Source: CAD feature listing. Evaluate the final solid. Frame: model axes, mm. A direction names the side the tool comes from. Round coordinates to 2 decimals unless told otherwise and drop trailing zeros. Loops run counter-clockwise (first coordinate to the right, second up) from the corner with the lowest first, then second, coordinate; pieces in that order, holes last. Notation, with made-up numbers: M 15,65 L 59,65 A10 ccw 59,71 Z; hole C 6.5,-37 d11. An arc over 180 degrees is marked long. One line per item, written item: value.
from build123d import *

# Parameters (mm, degrees)
SKETCH_1_W                      = 70
SKETCH_1_H                      = 105
EXTRUDE_1_DEPTH                 = 5
SKETCH_2_W                      = 30
SKETCH_2_H                      = 30
EXTRUDE_2_DEPTH                 = 120
EXTRUDE_3_REACH                 = 137.577
EXTRUDE_3_DIRECTION_2_REACH     = 137.577
SKETCH_8_R                      = 4.1
CUT_EXTRUDE_2_DEPTH             = 5
SKETCH_11_W                     = 20
SKETCH_11_H                     = 105
CUT_EXTRUDE_3_DEPTH             = 5
PATTERN_LINEAR_1_COUNT          = 3
PATTERN_LINEAR_1_PITCH          = 45.6
CUT_EXTRUDE_4_DEPTH             = 9
CUT_EXTRUDE_4_DEPTH_BACK        = 136.57746863
SKETCH_14_W                     = 13.2
SKETCH_14_H                     = 24
PATTERN_LINEAR_3_COUNT          = 2
PATTERN_LINEAR_3_PITCH          = 30
SKETCH_15_W                     = 30
SKETCH_15_H                     = 8.2
CUT_EXTRUDE_5_DEPTH             = 5
MIRROR_4_COPY_1_SKETCH_R        = 4.1
MIRROR_4_COPY_1_DEPTH           = 5
MIRROR_4_COPY_2_SKETCH_R        = 4.1
MIRROR_4_COPY_2_DEPTH           = 5
CUT_EXTRUDE_6_REACH             = 137.577
SKETCH_17_W                     = 13.2
SKETCH_17_H                     = 18
CUT_EXTRUDE_6_DIRECTION_2_DEPTH = 9
CUT_EXTRUDE_7_DEPTH             = 9
CUT_EXTRUDE_7_DEPTH_BACK        = 15
SKETCH_18_W                     = 13.2
SKETCH_18_H                     = 15


with BuildPart() as part:
    # 草图1 → 凸台-拉伸1 (new body)
    with BuildSketch(Plane(origin=(0, 0, 0), x_dir=(1, 0, 0), z_dir=(0, 1, 0))):
        Rectangle(SKETCH_1_W, SKETCH_1_H)
    extrude(amount=EXTRUDE_1_DEPTH)

    # 草图2 → 凸台-拉伸2 (add)
    with BuildSketch(Plane(origin=(0, 0, 0), x_dir=(1, 0, 0), z_dir=(0, 1, 0))):
        Rectangle(SKETCH_2_W, SKETCH_2_H)
    extrude(amount=EXTRUDE_2_DEPTH)

    # 凸台-拉伸3: up to this face of the body (flat: up to its plane)
    extrude_3_end = Plane(part.part.faces().sort_by_distance((0, 62.5, 15))[0])
    # 草图7 → 凸台-拉伸3 (add, up to the picked face)
    with BuildSketch(Plane.XY, mode=Mode.PRIVATE) as extrude_3_sk1:
        Polygon((-15, 25), (-35, 5), (-15, 5), align=None)
    extrude_3_tool1 = split(extrude(extrude_3_sk1.sketch, amount=EXTRUDE_3_REACH, mode=Mode.PRIVATE), bisect_by=extrude_3_end, keep=Keep.BOTH, mode=Mode.PRIVATE)
    add(extrude_3_tool1.solids().sort_by(Axis((-21.666667, 11.666667, 0), (0, 0, 1)))[0])

    # 凸台-拉伸3 direction 2: up to this face of the body (flat: up to its plane)
    extrude_3_direction_2_end = Plane(part.part.faces().sort_by_distance((0, 62.5, -15))[0])
    # 草图7 → 凸台-拉伸3 direction 2 (add, up to the picked face)
    with BuildSketch(Plane.XY, mode=Mode.PRIVATE) as extrude_3_direction_2_sk1:
        Polygon((-15, 25), (-35, 5), (-15, 5), align=None)
    extrude_3_direction_2_tool1 = split(extrude(extrude_3_direction_2_sk1.sketch, amount=-EXTRUDE_3_DIRECTION_2_REACH, mode=Mode.PRIVATE), bisect_by=extrude_3_direction_2_end, keep=Keep.BOTH, mode=Mode.PRIVATE)
    add(extrude_3_direction_2_tool1.solids().sort_by(Axis((-21.666667, 11.666667, 0), (0, 0, -1)))[0])

    # 草图8 → 切除-拉伸2 (cut)
    with BuildSketch(Plane(origin=(0, 0, 0), x_dir=(1, 0, 0), z_dir=(0, 1, 0))):
        with Locations(Location((-25, 45, 0), (0, 0, 270))):
            Circle(SKETCH_8_R)
    cut_extrude_2 = extrude(amount=CUT_EXTRUDE_2_DEPTH, mode=Mode.SUBTRACT)

    # 镜向2: 切除-拉伸2 across plane
    add(cut_extrude_2.mirror(Plane.XY), mode=Mode.SUBTRACT)

    # 草图11 → 切除-拉伸3 (cut)
    with BuildSketch(Plane(origin=(0, 0, 0), x_dir=(1, 0, 0), z_dir=(0, 1, 0))):
        with Locations((25, 0)):
            Rectangle(SKETCH_11_W, SKETCH_11_H)
    extrude(amount=CUT_EXTRUDE_3_DEPTH, mode=Mode.SUBTRACT)

    # 草图12 → 切除-旋转2 (revolve, cut)
    with BuildSketch(Plane.XY):
        with BuildLine():
            Line((15, 20), (15, 0))
            ThreePointArc((15, 0), (5, 10), (15, 20))
        make_face()
    cut_revolve_2 = revolve(axis=Axis((15, 20, 0), (0, -1, 0)), mode=Mode.SUBTRACT)

    # 阵列(线性)1: 切除-旋转2 ×3
    with Locations(*[(0, i * PATTERN_LINEAR_1_PITCH, 0) for i in range(1, PATTERN_LINEAR_1_COUNT)]):
        add(cut_revolve_2, mode=Mode.SUBTRACT)

    # 草图14 → 切除-拉伸4 (cut, two sides: drawn at the far end of the back side and taken through both)
    with BuildSketch(Plane(origin=(0, 0, 0), x_dir=(0, 0, -1), z_dir=(1, 0, 0)).offset(-CUT_EXTRUDE_4_DEPTH_BACK)):
        with Locations((0.067878733, 103.977253559)):
            Rectangle(SKETCH_14_W, SKETCH_14_H)
    extrude(amount=CUT_EXTRUDE_4_DEPTH + CUT_EXTRUDE_4_DEPTH_BACK, mode=Mode.SUBTRACT)

    # 阵列(线性)3: 切除-拉伸2 ×2
    with Locations(*[(i * PATTERN_LINEAR_3_PITCH, 0, 0) for i in range(1, PATTERN_LINEAR_3_COUNT)]):
        add(cut_extrude_2, mode=Mode.SUBTRACT)

    # 草图15 → 切除-拉伸5 (cut)
    with BuildSketch(Plane(origin=(0, 0, 0), x_dir=(1, 0, 0), z_dir=(0, 1, 0))):
        with Locations((-10, 45)):
            Rectangle(SKETCH_15_W, SKETCH_15_H)
    cut_extrude_5 = extrude(amount=CUT_EXTRUDE_5_DEPTH, mode=Mode.SUBTRACT)

    # 镜向3: 切除-拉伸5 across plane
    add(cut_extrude_5.mirror(Plane.XY), mode=Mode.SUBTRACT)

    # 镜向4 copy 1 sketch → 镜向4 copy 1 (cut)
    with BuildSketch(Plane(origin=(30, 0, 0), x_dir=(1, 0, 0), z_dir=(0, 1, 0))):
        with Locations((-25, -45)):
            Circle(MIRROR_4_COPY_1_SKETCH_R)
    extrude(amount=MIRROR_4_COPY_1_DEPTH, mode=Mode.SUBTRACT)

    # 镜向4 copy 2 sketch → 镜向4 copy 2 (cut)
    with BuildSketch(Plane(origin=(0, 0, 0), x_dir=(1, 0, 0), z_dir=(0, 1, 0))):
        with Locations((-25, -45)):
            Circle(MIRROR_4_COPY_2_SKETCH_R)
    extrude(amount=MIRROR_4_COPY_2_DEPTH, mode=Mode.SUBTRACT)

    # 切除-拉伸6: up to this plane
    cut_extrude_6_end = Plane(origin=(-15, 25, 43.284271247), z_dir=(0.7071067811865476, -0.7071067811865475, 0))
    # 草图17 → 切除-拉伸6 (cut, up to the surface)
    with BuildSketch(Plane(origin=(0, 0, 0), x_dir=(0, 0, -1), z_dir=(1, 0, 0)), mode=Mode.PRIVATE) as cut_extrude_6_sk1:
        with Locations((0, 9)):
            Rectangle(SKETCH_17_W, SKETCH_17_H)
    cut_extrude_6_tool1 = split(extrude(cut_extrude_6_sk1.sketch, amount=-CUT_EXTRUDE_6_REACH, mode=Mode.PRIVATE), bisect_by=cut_extrude_6_end, keep=Keep.BOTH, mode=Mode.PRIVATE)
    add(cut_extrude_6_tool1.solids().sort_by_distance((0, 9, 0))[0], mode=Mode.SUBTRACT)

    # 草图17 → 切除-拉伸6 direction 2 (cut)
    with BuildSketch(Plane(origin=(0, 0, 0), x_dir=(0, 0, -1), z_dir=(1, 0, 0))):
        with Locations((0, 9)):
            Rectangle(SKETCH_17_W, SKETCH_17_H)
    extrude(amount=CUT_EXTRUDE_6_DIRECTION_2_DEPTH, mode=Mode.SUBTRACT)

    # 草图18 → 切除-拉伸7 (cut, two sides: drawn at the far end of the back side and taken through both)
    with BuildSketch(Plane(origin=(0, 0, 0), x_dir=(0, 0, -1), z_dir=(1, 0, 0)).offset(-CUT_EXTRUDE_7_DEPTH_BACK)):
        with Locations((0.014378278, 55.6)):
            Rectangle(SKETCH_18_W, SKETCH_18_H)
    extrude(amount=CUT_EXTRUDE_7_DEPTH + CUT_EXTRUDE_7_DEPTH_BACK, mode=Mode.SUBTRACT)


solid = part.part
1. Reachability of faces 4 (the face through (9, 17, 5)), 5 (the face through (1, 63, 15)), 6 (the face through (9.1, 2.5, 45.1)), 7 (the face through (9, 62, 6)) from +Z, -Z, +X, -X, +Y, -Y: full face, straight path, thin tool, end or side. Return the list, or none.
Report:
face 4: -X, -Y
face 5: +Z, +X, -X, +Y
face 6: +Y, -Y
face 7: -X
2. Section query B-B (z = 45). Return the cut outline in (x, y), and give its area (3 significant figures).
Report:
outline: M -35,0 L -29.1,0 L -29.1,5 L -35,5 Z; M 9.1,0 L 15,0 L 15,5 L 9.1,5 Z
area: 59.0 mm2
3. Section query D-D (z = -4.5). Return the cut outline in (x, y), and give its area (3 significant figures).
Report:
outline: M -22,18 L 9,18 L 9,16.61 A8.93 cw 15,18.93 L 15,46.67 A8.93 cw 9,48.99 L 9,48.1 L -15,48.1 L -15,25 Z; M -15,63.1 L 9,63.1 L 9,62.21 A8.93 cw 15,64.53 L 15,92.27 A8.93 cw 9,94.59 L 9,91.98 L -15,91.98 Z; M -15,115.98 L 9,115.98 L 9,107.81 A8.93 cw 15,110.13 L 15,120 L -15,120 Z; M 9,0 L 15,0 L 15,1.07 A8.93 cw 9,3.39 Z
area: 1,960 mm2
4. Pin query (flat end, axial travel): pin 1 (2.5 mm diameter, centred on y = 61, z = -5.5, fed in from -X); pin 2 (6 mm diameter, centred on x = -21.5, z = 15, fed in from +Y); pin 3 (1.6 mm diameter, centred on y = 2.5, z = 3, fed in from -X). Return the tip coordinate at first contact, or that it passes through.
Report:
pin 1: stops at x = -15
pin 2: stops at y = 21.5
pin 3: stops at x = 9
5. Ray query, line 1 (Z direction, x = 6.5, y = 62); line 2 (Z direction, x = -9.5, y = 109); line 3 (Y direction, x = -24, z = -33). Return the intervals inside material, ascending. Write a range as [from, to].
Report:
line 1: z = [-15, -6.61], [6.59, 15]
line 2: z = [-15, -6.67], [6.53, 15]
line 3: y = [0, 5]
6. Pull-direction query (Y, two-part tool) for faces 1 (the face through (-20, 20, 0)), 2 (the face through (-6, 18, 0)), 3 (the face through (-3, 104, -6.668)); classes: released by +Y, released by -Y, zero draft, split by the parting line, or undercut.
Report:
face 1: released by +Y
face 2: released by -Y
face 3: undercut
7. Section query A-A (x = -11). Return the cut outline in (y, z), and give its area (3 significant figures).
Report:
outline: M 0,-52.5 L 5,-52.5 L 5,-49.1 L 0,-49.1 Z; M 0,-40.9 L 5,-40.9 L 5,-15 L 120,-15 L 120,15 L 5,15 L 5,40.9 L 0,40.9 L 0,6.6 L 18,6.6 L 18,-6.6 L 0,-6.6 Z; M 0,49.1 L 5,49.1 L 5,52.5 L 0,52.5 Z; hole M 48.1,-6.61 L 63.1,-6.61 L 63.1,6.59 L 48.1,6.59 Z; hole M 91.98,-6.67 L 115.98,-6.67 L 115.98,6.53 L 91.98,6.53 Z
area: 3,140 mm2
8. Section query C-C (y = 100). Return the cut outline in (x, z), and give its area (3 significant figures).
Report:
outline: M -15,-15 L 15,-15 L 15,-9.93 A9.93 cw 7.64,-6.67 L -15,-6.67 Z; M -15,6.53 L 7.52,6.53 A9.93 cw 15,9.93 L 15,15 L -15,15 Z
area: 470 mm2
